Can you work these out from the drawing? Everything is in mm from the part's minimum corner. Give positions to 0.01 mm unless a question says otherwise; leave off trailing zeros. Order: outer loops, then holes, each group sorted by start corner. A loop starts at its lowest first (then second) coordinate and runs counter-clockwise, first axis right, second up. Notation, with made-up numbers: M -22,28 L -12,28 A22 cw -12,67 Z; hole C -26,67.25 d1. An arc over 180 degrees is marked long. Answer as a JSON object with one key per item and string values.
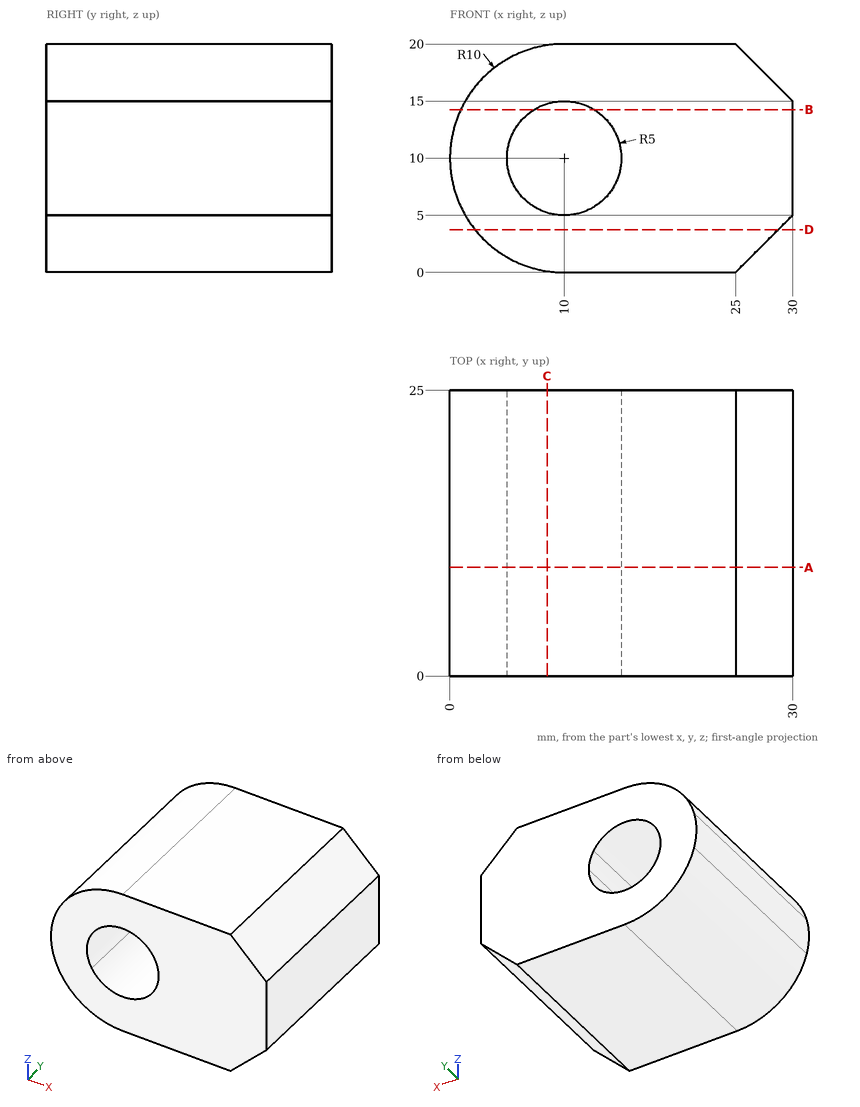
1) I need wall thicknesses on L1, parallel to Z at x = 12.5, y = 13.75; L2, parallel to Z at x = 8.25, y = 23.5; L3, parallel to X at y = 3.25, z = 14.25. Which ranges of each line are inside material? Lowest first, please.
Results found:
{"L1": "z = 0 to 5.67, 14.33 to 20", "L2": "z = 0.15 to 5.32, 14.68 to 19.85", "L3": "x = 0.95 to 7.37, 12.63 to 30"}
2) I want a section at B-B on z = 14.25. Write out the boundary of the cut face in (x, y).
Results found:
{"outline": "M 0.95,0 L 7.37,0 L 7.37,25 L 0.95,25 Z; M 12.63,0 L 30,0 L 30,25 L 12.63,25 Z"}
3) I want a section at A-A on y = 9.5. Write out the boundary of the cut face in (x, z), and give its area (3 significant figures).
Results found:
{"outline": "M 0.32,7.5 A10 ccw 10,0 L 25,0 L 30,5 L 30,15 L 25,20 L 10,20 A10 ccw 0.32,12.5 A10 ccw Z; hole M 14.33,7.5 A5 ccw 15,10 A5 ccw 14.33,12.5 A5 ccw long Z", "area": "454 mm²"}
4) I want a section at D-D on z = 3.75. Write out the boundary of the cut face in (x, y).
Results found:
{"outline": "M 2.19,0 L 28.75,0 L 28.75,25 L 2.19,25 Z"}
5) I'm going to push flat-ended pins straight in: pin 1 Ø3 at (y, z) = (9.5, 3) entering from -X; pin 2 Ø1.5 at (x, y) = (4.5, 18.5) entering from +Z; pin 3 Ø2 at (x, z) = (13, 8) entering from -Y; pin 4 Ø12 at (x, z) = (20, 8.5) entering from -Y. Where does each tip first touch, or does it pass through?
Results found:
{"pin 1": "stops at x = 1.65", "pin 2": "stops at z = 18.8", "pin 3": "passes through", "pin 4": "stops at y = 0"}
6) I want a section at C-C on x = 8.5. Write out the boundary of the cut face in (y, z).
Results found:
{"outline": "M 0,0.11 L 25,0.11 L 25,5.23 L 0,5.23 Z; M 0,14.77 L 25,14.77 L 25,19.89 L 0,19.89 Z"}
